Input: part model. Units: mm. Frame: model coordinates. A direction names the side the tool comes from. Coordinates: 2 decimals unless noted, no trailing zeros. Order: outer loops, then holes, each group sorted by start corner. A loop starts at its lowest first (then second) coordinate and runs counter-clockwise, first axis right, second up. Notation, with made-up numbers: M 81.5,54 L 91.5,54 A27 ccw 91.5,84 Z; hole C 0.25,-34 d5. An arc over 180 degrees is marked long. One line per item, written item: value.
```python
from build123d import *

# Parameters (mm, degrees)
SKETCH1_W           = 10
SKETCH1_H           = 25
SKETCH1_R           = 1.7
BOSS_EXTRUDE1_DEPTH = 5
SKETCH2_W           = 25
SKETCH2_H           = 25
SKETCH2_W_2         = 5
BOSS_EXTRUDE2_DEPTH = 5
SKETCH3_R           = 3.95
BOSS_EXTRUDE3_DEPTH = 3
SKETCH4_R           = 3
CUT_EXTRUDE1_DEPTH  = 3
FILLET1_R           = 12.5
BOSS_EXTRUDE4_DEPTH = 1.5
FILLET2_R           = 5


# Some blends are built 0.0001 mm under size
with BuildPart() as part:
    # Sketch1 → Boss-Extrude1 (new body)
    with BuildSketch(Plane.XY):
        with Locations((259.023766163, 223.42362241)):
            Rectangle(SKETCH1_W, SKETCH1_H)
        with Locations((259.023766163, 229.92362241)):
            Circle(SKETCH1_R, mode=Mode.SUBTRACT)
        with Locations((259.023766163, 216.92362241)):
            Circle(SKETCH1_R, mode=Mode.SUBTRACT)
    extrude(amount=BOSS_EXTRUDE1_DEPTH)

    # Sketch2 → Boss-Extrude2 (add)
    with BuildSketch(Plane.ZY.offset(-254.023766163)):
        with Locations((17.5, 223.42362241)):
            Rectangle(SKETCH2_W, SKETCH2_H)
        with Locations((2.5, 223.42362241)):
            Rectangle(SKETCH2_W_2, SKETCH2_H)
    extrude(amount=BOSS_EXTRUDE2_DEPTH)

    # Sketch3 → Boss-Extrude3 (add)
    with BuildSketch(Plane.ZY.offset(-249.023766163)):
        with Locations((17.5, 223.42362241)):
            Circle(SKETCH3_R)
    extrude(amount=BOSS_EXTRUDE3_DEPTH)

    # Sketch4 → Cut-Extrude1 (cut)
    with BuildSketch(Plane.XY.offset(5)):
        with Locations((259.023766163, 216.92362241)):
            Circle(SKETCH4_R)
        with Locations((259.023766163, 229.92362241)):
            Circle(SKETCH4_R)
    extrude(amount=-CUT_EXTRUDE1_DEPTH, mode=Mode.SUBTRACT)

    # Fillet1
    fillet1_edges = [part.edges().sort_by_distance(p)[0] for p in [
        (251.523766163, 210.92362241, 30),
        (251.523766163, 235.92362241, 30),
    ]]
    fillet(fillet1_edges, radius=FILLET1_R - 0.0001)  # a hair under: the kernel refuses the full size

    # Sketch5 → Boss-Extrude4 (add, symmetric)
    with BuildSketch(Plane(origin=(0, 223.42362241, 0), x_dir=(1, 0, 0), z_dir=(0, 1, 0))):
        Polygon((254.023766163, -28.1700362), (264.023766163, -5), (254.023766163, -5), (254.023766163, -17.5), align=None)
    extrude(amount=BOSS_EXTRUDE4_DEPTH, both=True)

    # Fillet2
    # the kernel refuses this fillet: 5 mm, written as the material it adds along each edge
    with BuildSketch(Plane(origin=(254.023766163, 235.92362241, 5), x_dir=(0, 0, 1), z_dir=(0, -1, 0))) as fillet2_piece_1_section:
        with BuildLine():
            CenterArc((FILLET2_R, -FILLET2_R), FILLET2_R, 90, 90)
            Line((0, -FILLET2_R), (0, 0))
            Line((0, 0), (FILLET2_R, 0))
        make_face()
    fillet2_piece_1 = extrude(amount=23.5, mode=Mode.PRIVATE)
    fillet2_piece_1 = fillet2_piece_1 - Plane(origin=(259.023766163, 229.92362241, 6.20300882), x_dir=(1, 0, 0), z_dir=(0, 0, 1)) * Cylinder(3, 68, mode=Mode.PRIVATE)
    fillet2_piece_1 = fillet2_piece_1 - Plane(origin=(259.023766163, 216.92362241, 6.20300882), x_dir=(1, 0, 0), z_dir=(0, 0, 1)) * Cylinder(3, 68, mode=Mode.PRIVATE)
    add(fillet2_piece_1)
    with BuildSketch(Plane(origin=(254.023766163, 234.42362241, 5), x_dir=(0, 0, 1), z_dir=(0, -1, 0))) as fillet2_piece_2_section:
        with BuildLine():
            CenterArc((FILLET2_R, -FILLET2_R), FILLET2_R, 90, 90)
            Line((0, -FILLET2_R), (0, 0))
            Line((0, 0), (FILLET2_R, 0))
        make_face()
    fillet2_piece_2 = extrude(amount=23.5, mode=Mode.PRIVATE)
    fillet2_piece_2 = fillet2_piece_2 - Plane(origin=(259.023766163, 229.92362241, 6.193943695), x_dir=(1, 0, 0), z_dir=(0, 0, 1)) * Cylinder(3, 67, mode=Mode.PRIVATE)
    fillet2_piece_2 = fillet2_piece_2 - Plane(origin=(259.023766163, 216.92362241, 6.193943695), x_dir=(1, 0, 0), z_dir=(0, 0, 1)) * Cylinder(3, 67, mode=Mode.PRIVATE)
    add(fillet2_piece_2)


solid = part.part
```
(1) Cut plane B-B on y = 234. Output: boundary loops of the cut face in (x, z).
Data:
outline: M 249.02,0 L 264.02,0 L 264.02,5 L 259.02,5 A5 cw 254.02,10 L 254.02,24.16 L 249.02,24.16 Z
(2) Draft query along Y for faces 1 (the flat face through (255, 210.924, 6.7)), 2 (the flat face through (246.024, 223, 17)), 3 (the flat face through (259, 228, 2)), 4 (the flat face through (259, 215, 2)). Return one class per face: released by +Y, released by -Y, zero draft, split by the parting line, or undercut.
Data:
face 1: released by -Y
face 2: zero draft
face 3: undercut
face 4: undercut
(3) Cut plane C-C on z = 5.5. Output: boundary loops of the cut face in (x, y), plus the area to 3 significant figures.
Data:
outline: M 249.02,210.92 L 256.84,210.92 L 256.84,214.86 A3 cw 256.84,218.99 L 256.84,221.92 L 263.81,221.92 L 263.81,224.92 L 256.84,224.92 L 256.84,227.86 A3 cw 256.84,231.99 L 256.84,235.92 L 249.02,235.92 Z
area: 212 mm2
(4) Cut plane D-D on y = 220.75. Output: boundary loops of the cut face in (x, z).
Data:
outline: M 246.02,14.59 L 249.02,14.59 L 249.02,0 L 264.02,0 L 264.02,5 L 259.02,5 A5 cw 254.02,10 L 254.02,29.71 L 249.02,29.71 L 249.02,20.41 L 246.02,20.41 Z
(5) Cut plane A-A on z = 22.5. Output: boundary loops of the cut face in (x, y), plus the area to 3 significant figures.
Data:
outline: M 249.02,211.97 L 254.02,211.97 L 254.02,221.92 L 256.47,221.92 L 256.47,224.92 L 254.02,224.92 L 254.02,234.88 L 249.02,234.88 Z
area: 122 mm2
(6) Ray query, line 1 (Y direction, x = 254.25, z = 27.5); line 2 (X direction, y = 227.75, z = 10.5); line 3 (X direction, y = 217.5, z = 6). Return the intervals inside material, ascending. Write a range as from..to.
Data:
line 1: y = 221.92..224.92
line 2: x = 249.02..254.02
line 3: x = 249.02..256.02
(7) Access query for faces 5 (the flat face through (254.024, 221, 20)), 6 (the cylindrical face through (247.54, 219.92, 19.32)), 7 (the flat face through (263, 217, 5)), 8 (the flat face through (262, 231, 5)). Directions: +Z, -Z, +X, -X, +Y, -Y. A direction counts if a zero-diameter tool reaches every point of the face in a straight line with its end or side. Return the directions, or none.
Data:
face 5: +Z, +X
face 6: -X
face 7: +Z, +X, -Y
face 8: +Z, +X, +Y
(8) First-contact query: pin 1 (5.5 mm diameter, centred on x = 259.02, y = 216.92, fed in from +Z); pin 2 (4 mm diameter, centred on x = 261, y = 232.5, fed in from +Z); pin 3 (2 mm diameter, centred on y = 228.5, z = 19, fed in from +X); pin 4 (8 mm diameter, centred on x = 256.5, z = 13, fed in from -Y). Flat tips, straight axial feed; report the tip coordinate or a pass-through.
Data:
pin 1: stops at z = 2
pin 2: stops at z = 5
pin 3: stops at x = 254.02
pin 4: stops at y = 210.92
